```python
from build123d import *

# Parameters (mm, degrees)
SKETCH1_R           = 5
SKETCH1_W           = 6.35
SKETCH1_H           = 6.35
BOSS_EXTRUDE1_DEPTH = 3.175
FILLET1_R           = 0.635


with BuildPart() as part:
    # Sketch1 → Boss-Extrude1 (new body)
    with BuildSketch(Plane(origin=(0, 0, 0), x_dir=(0, 0, -1), z_dir=(1, 0, 0))):
        Circle(SKETCH1_R)
        Rectangle(SKETCH1_W, SKETCH1_H, mode=Mode.SUBTRACT)
    extrude(amount=BOSS_EXTRUDE1_DEPTH)

    # Fillet1
    fillet1_edges = [part.edges().sort_by_distance(p)[0] for p in [
        (1.5875, -3.175, 3.175),
        (1.5875, -3.175, -3.175),
        (1.5875, 3.175, -3.175),
        (1.5875, 3.175, 3.175),
    ]]
    fillet(fillet1_edges, radius=FILLET1_R)


solid = part.part
```
Verification items for the finished model (mm, model axes). Coordinates: 2 decimals unless noted, no trailing zeros. Loops run counter-clockwise (first coordinate to the right, second up) from the corner with the lowest first, then second, coordinate; pieces in that order, holes last. Notation, with made-up numbers: (-29, 58.5) -> (12, 58.5) arc R30 ccw to (12, 93.5) -> close; hole circle Ø11 at (17, -24). An arc over 180 degrees is marked (long way). Put each result on its own line as item: value.
1. Section check C-C, the plane z = -1.5. Record the boundary of the cut face in (x, y) (3 decimals).
Result set:
outline: (0, -4.77) -> (3.175, -4.77) -> (3.175, -3.175) -> (0, -3.175) -> close; (0, 3.175) -> (3.175, 3.175) -> (3.175, 4.77) -> (0, 4.77) -> close
2. Section check B-B, the plane x = 0.7. Record the boundary of the cut face in (y, z) (3 decimals), then the cut area to 3 significant figures.
Result set:
outline: circle Ø10 at (0, 0); hole (-3.175, -2.54) arc R0.635 ccw to (-2.54, -3.175) -> (2.54, -3.175) arc R0.635 ccw to (3.175, -2.54) -> (3.175, 2.54) arc R0.635 ccw to (2.54, 3.175) -> (-2.54, 3.175) arc R0.635 ccw to (-3.175, 2.54) -> close
area: 38.6 mm^2
3. Thickness scan on line 1 (Z direction, x = 1.6, y = 1.75) (3 decimals); line 2 (Y direction, x = 1.3, z = -1.25) (3 decimals). Record the ranges inside material, lowest first.
Result set:
line 1: z = -4.684 to -3.175, 3.175 to 4.684
line 2: y = -4.841 to -3.175, 3.175 to 4.841
4. Section check D-D, the plane z = -4.25. Record the boundary of the cut face in (x, y) (3 decimals), then the cut area to 3 significant figures.
Result set:
outline: (0, -2.634) -> (3.175, -2.634) -> (3.175, 2.634) -> (0, 2.634) -> close
area: 16.7 mm^2
5. Mould release check, pull along Z, two halves, no side actions. Record for faces 1 (the face through (1.57, -4.88, 1.08)), 2 (the face through (2, 3.175, 0)): pulls with the +Z half, pulls with the -Z half, needs draft (parallel to the pull), parting line crosses it, or undercut.
Result set:
face 1: parting line crosses it
face 2: undercut
6. Section check A-A, the plane y = 0. Record the boundary of the cut face in (x, z) (3 decimals), then the cut area to 3 significant figures.
Result set:
outline: (0, -5) -> (3.175, -5) -> (3.175, -3.175) -> (0, -3.175) -> close; (0, 3.175) -> (3.175, 3.175) -> (3.175, 5) -> (0, 5) -> close
area: 11.6 mm^2
7. Gauge pin test, flat ends, axial feed: P1, Ø1.6, axis at x = 2, z = 0.5, coming from the +Y side; P2, Ø1.6, axis at x = 2, y = 1, coming from the +Z side; P3, Ø1.5, axis at y = 2, z = -2, coming from the +X side. Record the tip position at first contact, or that the pin passes through.
Result set:
P1: stops at y = 5
P2: stops at z = 5
P3: passes through
